Autodesk Inventor part; units mm, degrees
ref_plane "YZ Plane" through (0, 0, 0) normal (1, 0, 0) x (0, 1, 0)
ref_plane "XZ Plane" through (0, 0, 0) normal (0, 1, 0) x (-1, 0, 0)
ref_plane "XY Plane" through (0, 0, 0) normal (0, 0, 1) x (1, 0, 0)
sketch "Sketch1" plane through (0, 0, 0) normal (0, 0, 1) x (1, 0, 0)
  circle A0 centre (0, 0) radius 5.715
  circle A1 centre (0, 0) radius 15.875 construction
  circle A2 centre (0, 15.875) radius 3.175
  circle A3 centre (0, -15.875) radius 3.175
  circle A4 centre (0, 0) radius 11.1125
  line L0 (0, 15.875) -> (0, -15.875) construction
  line L1 (-3.175, 15.875) -> (-3.175, -15.875)
  line L2 (3.175, -15.875) -> (3.175, 15.875)
  arc A5 (3.175, 15.875) -> (-3.175, 15.875) centre (0, 15.875) ccw
  arc A6 (-3.175, -15.875) -> (3.175, -15.875) centre (0, -15.875) ccw
  circle A7 centre (0, -7.366) radius 0.8255
  circle A8 centre (0, 0) radius 7.366 construction
  circle A9 centre (5.2085, -5.2085) radius 0.8255
  circle A10 centre (-5.2085, -5.2085) radius 0.8255
  point P0 (-3.175, 10.6493)
  point P1 (-3.175, -10.6493)
  point P2 (3.175, -10.6493)
  point P3 (3.175, 10.6493)
  point P4 (3.175, 15.875)
  point P5 (3.175, -15.875)
  dimension "d0" = 11.43
  dimension "d1" = 31.75
  dimension "d2" = 6.35
  dimension "d3" = 22.225
  dimension "d6" = 1.651
  dimension "d12" = 14.732
  dimension "d13" = 45
  dimension "d14" = 45
extrude "Extrusion1" add sketch "Sketch1" along normal blind 3.175 contours A0 L2 A4 | A0 L1 A4 L2 | L2 A4 L1 A0 | A0 L1 A4 | A4 L1 A2 L2 | L2 A3 L1 A4 | A2 | A3
extrude "Extrusion2" add sketch "Sketch1" against normal blind 3.175 contours A2 | A3
fillet "Fillet1" radius 3.175 4 edges at (-3.175, -10.6493, 1.5875) (3.175, -10.6493, 1.5875) (-3.175, 10.6493, 1.5875) (3.175, 10.6493, 1.5875)
properties part number "EncoderPinRetainer" material "ABS Plastic"
Source: CAD feature listing. Evaluate the final solid. Frame: model axes, mm. A direction names the side the tool comes from. Coordinates: 2 decimals unless noted, no trailing zeros. Write each loop counter-clockwise with the first axis right and the second up, starting at its lowest first coordinate (ties: lowest second). Pieces come first, ordered by that corner, then holes. Notation, with made-up numbers: M -31,65.25 L -17,65.25 A13 ccw -17,84.25 Z; hole C 89,12.5 d2. An arc over 180 degrees is marked long. Use a Markdown table: item, result.
1) First-contact query: pin 1 Ø3.5 at (y, z) = (14.5, 1.5) entering from +X; pin 2 Ø3 at (x, y) = (-2.5, 6) entering from -Z; pin 3 Ø2.5 at (y, z) = (-13.5, 1) entering from -X. Flat tips, straight axial feed; report the tip coordinate or a pass-through.
Conclusion:
| item | result |
|---|---|
| pin 1 | stops at x = 3.18 |
| pin 2 | stops at z = 0 |
| pin 3 | stops at x = -3.22 |
2) Section D-D, the plane z = -1. Output: boundary loops of the cut face in (x, y) (3 decimals), then the cut area to 3 significant figures.
Conclusion:
| item | result |
|---|---|
| outline | C 0,-15.875 d6.35; C 0,15.875 d6.35 |
| area | 63.3 mm^2 |
3) Ray query, L1, parallel to Y at x = 4.5, z = 1.5; L2, parallel to X at y = 0, z = 2.25 (1 decimal); L3, parallel to X at y = 15, z = 1.5 (3 decimals). Return the intervals inside material, ascending.
Conclusion:
| item | result |
|---|---|
| L1 | y = -10.22 to -5.63, -4.78 to -3.52, 3.52 to 10.22 |
| L2 | x = -11.1 to -5.7, 5.7 to 11.1 |
| L3 | x = -3.175 to 3.175 |
4) Section A-A, the plane x = 0. Give the number of separate pieces and of enclosed holes in the cut face, then the cut area to 3 significant figures.
Conclusion:
| item | result |
|---|---|
| separate pieces | 3 |
| enclosed holes | 0 |
| area | 120 mm^2 |
5) Section C-C, the plane x = 2.25. Output: boundary loops of the cut face in (y, z) (3 decimals).
Conclusion:
| item | result |
|---|---|
| outline | M -18.115,-3.175 L -13.635,-3.175 L -13.635,0 L -5.253,0 L -5.253,3.175 L -18.115,3.175 Z; M 5.253,0 L 13.635,0 L 13.635,-3.175 L 18.115,-3.175 L 18.115,3.175 L 5.253,3.175 Z |
6) Mould query, pull axis X, two halves, no side actions, for faces 6 (the cylindrical face through (-5.817, -5.766, 1.565)), 7 (the cylindrical face through (-3.665, 11.105, 1.61)), 8 (the flat face through (0, 16, -3.175)). Classes: pulls with the +X half, pulls with the -X half, needs draft (parallel to the pull), parting line crosses it, or undercut.
Conclusion:
| item | result |
|---|---|
| face 6 | undercut |
| face 7 | pulls with the -X half |
| face 8 | needs draft |
7) Section B-B, the plane y = 0. Output: boundary loops of the cut face in (x, z) (1 decimal), then the cut area to 3 significant figures.
Conclusion:
| item | result |
|---|---|
| outline | M -11.1,0 L -5.7,0 L -5.7,3.2 L -11.1,3.2 Z; M 5.7,0 L 11.1,0 L 11.1,3.2 L 5.7,3.2 Z |
| area | 34.3 mm^2 |
8) Reachability of faces 1 (the flat face through (-3.175, -14, 2)), 2 (the cylindrical face through (-0.688, 18.974, -0.75)), 3 (the flat face through (-3.175, 14, 2)), 4 (the flat face through (3.175, 14, 2)), 5 (the flat face through (3.175, -14, 2)) from +Z, -Z, +X, -X, +Y, -Y: full face, straight path, thin tool, end or side. Return the list, or none.
Conclusion:
| item | result |
|---|---|
| face 1 | +Z, -Z, -X, -Y |
| face 2 | -Z |
| face 3 | +Z, -Z, -X, +Y |
| face 4 | +Z, -Z, +X, +Y |
| face 5 | +Z, -Z, +X, -Y |
